The listing builds one solid part. Answer for the finished solid, in the listing's coordinates (mm). Face numbers are marked on the shaded views. Coordinates: 2 decimals unless noted, no trailing zeros. Write each loop counter-clockwise with the first axis right and the second up, starting at its lowest first coordinate (ties: lowest second). Pieces come first, ordered by that corner, then holes.
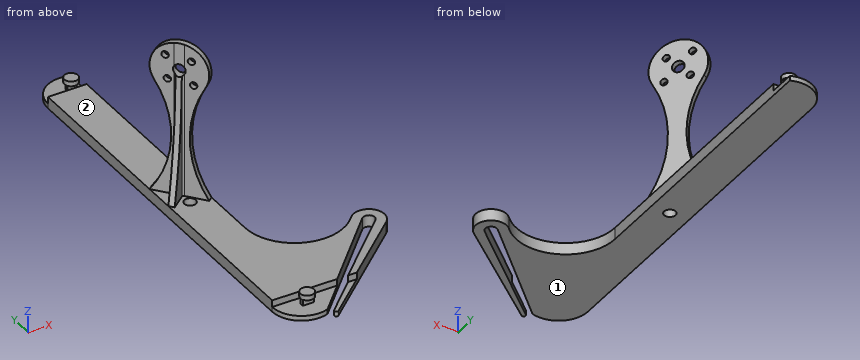
from build123d import *

# Parameters (mm, degrees)
PAD_DEPTH       = 6
SKETCH001_W     = 31.342523
SKETCH001_H     = 18.2690453429
SKETCH001_R     = 2.5
POCKET_DEPTH    = 3.5
SKETCH013_W     = 48.164109
SKETCH013_H     = 19.3260583096
SKETCH013_R     = 3.021402
POCKET008_DEPTH = 3.5
PAD001_DEPTH    = 80
POCKET009_DEPTH = 3
SKETCH015_R     = 3
SKETCH015_R_2   = 1.75
POCKET010_DEPTH = 80.3906309058
POCKET011_DEPTH = 5.5
POCKET012_DEPTH = 3.5
POCKET013_DEPTH = 3.5
SKETCH022_R     = 3.5
PAD002_DEPTH    = 2.5
SKETCH023_R     = 3.5
PAD003_DEPTH    = 2.5
SKETCH024_R     = 3
POCKET014_DEPTH = 6.001


with BuildPart() as part:
    # Sketch → Pad (new body)
    with BuildSketch(Plane.XY):
        with BuildLine():
            Line((148.7359710531, -99.0646793429), (148.7359710531, 92.9353206571))
            ThreePointArc((168.7359710531, 107.0774562808), (155.0757170152, 105.182769371), (148.7359710531, 92.9353206571))
            Line((168.7359710531, -42.6963517772), (168.7359710531, 107.0774562808))
            ThreePointArc((168.7359710531, -42.6963517772), (185.2022873789, -66.5007048599), (213.2847541452, -59.4891530095))
            ThreePointArc((224.5749857013, -70.7793845656), (224.9509601574, -59.1131785534), (213.2847541452, -59.4891530095))
            Line((172.271504959, -116.7423812201), (224.5749857013, -70.7793845656))
            ThreePointArc((170.8572913966, -115.3281676577), (170.8572913966, -116.7423812201), (172.271504959, -116.7423812201))
            Line((170.8572913966, -115.3281676577), (221.4154262515, -66.8913531464))
            ThreePointArc((221.4154262515, -66.8913531464), (221.4154262515, -62.6487124593), (217.1727855643, -62.6487124593))
            Line((168.7359710531, -113.2068473142), (217.1727855643, -62.6487124593))
            ThreePointArc((148.7359710531, -99.0646793429), (155.0757038094, -111.3121510664), (168.7359710531, -113.2068473142))
        make_face()
    extrude(amount=PAD_DEPTH)

    # Sketch001 → Pocket (cut)
    with BuildSketch(Plane.XY.offset(6)):
        with Locations((159.4964165, 102.0698433285)):
            Rectangle(SKETCH001_W, SKETCH001_H)
        with Locations((163.7359710531, 97.9353206571)):
            Circle(SKETCH001_R, mode=Mode.SUBTRACT)
    extrude(amount=-POCKET_DEPTH, mode=Mode.SUBTRACT)

    # Sketch013 → Pocket008 (cut)
    with BuildSketch(Plane.XY.offset(6)):
        with Locations((169.3588635, -108.7277408452)):
            Rectangle(SKETCH013_W, SKETCH013_H)
        with Locations((163.7359710531, -104.0647116904)):
            Circle(SKETCH013_R, mode=Mode.SUBTRACT)
    extrude(amount=-POCKET008_DEPTH, mode=Mode.SUBTRACT)

    # Sketch014 → Pad001 (new body)
    with BuildSketch(Plane.XY.offset(6)):
        with BuildLine():
            Line((148.7359710531, 5.9602104844), (155.9970967848, -3.0092063605))
            ThreePointArc((155.849066174, -4.4156511472), (156.2143657321, -3.7430868972), (155.9970967848, -3.0092063605))
            Line((148.7359710531, -10.174005219), (155.849066174, -4.4156511472))
            Line((148.7359710531, -10.174005219), (150.6235923171, -12.5057183154))
            Line((150.6235923171, -12.5057183154), (157.7366874381, -6.7473642436))
            ThreePointArc((159.1431322249, -6.8953948544), (158.4705679748, -6.5300952963), (157.7366874381, -6.7473642436))
            Line((159.1431322249, -6.8953948544), (166.4042579566, -15.8648116991))
            Line((166.4042579566, -15.8648116991), (168.7359710531, -13.9771904352))
            Line((151.0676841499, 7.8478317492), (168.7359710531, -13.9771904352))
            Line((148.7359710531, 5.9602104844), (151.0676841499, 7.8478317492))
        make_face()
    extrude(amount=PAD001_DEPTH)

    # Sketch016 → Pocket009 (cut)
    with BuildSketch(Plane(origin=(95.0976832559, 76.9856331596, 0), x_dir=(-0.629207088, 0.7772376988, 0), z_dir=(0.7772376988, 0.629207088, 0))):
        with BuildLine():
            ThreePointArc((-90.8226866435, 64.9598793146), (-102.9933476305, 86), (-115.1640086175, 64.9598793146))
            ThreePointArc((-117.0334683159, 6), (-107.9048310085, 35.2201328201), (-115.1640086175, 64.9598793146))
            Line((-117.0334683159, 6), (-129.946838, 10.190964))
            Line((-129.946838, 10.190964), (-129.946838, 98.716408))
            Line((-129.946838, 98.716408), (-69.304048, 98.716408))
            Line((-69.304048, 98.716408), (-45.866948, 9.880296))
            Line((-45.866948, 9.880296), (-88.9532269451, 6))
            ThreePointArc((-90.8226866435, 64.9598793146), (-99.1328607178, 35.18680854), (-88.9532269451, 6))
        make_face()
    extrude(amount=-POCKET009_DEPTH, mode=Mode.SUBTRACT)

    # Sketch015 → Pocket010 (cut, through all)
    with BuildSketch(Plane(origin=(95.0976832559, 76.9856331596, 0), x_dir=(-0.629207088, 0.7772376988, 0), z_dir=(0.7772376988, 0.629207088, 0))):
        with Locations((-102.9933476305, 71.9598793146)):
            Circle(SKETCH015_R)
        with Locations((-96.2758332092, 78.6773937359)):
            Circle(SKETCH015_R_2)
        with Locations((-108.65020188, 77.6167335641)):
            Circle(SKETCH015_R_2)
        with Locations((-109.7108620518, 65.2423648933)):
            Circle(SKETCH015_R_2)
        with Locations((-97.336493381, 66.3030250651)):
            Circle(SKETCH015_R_2)
    extrude(amount=-POCKET010_DEPTH, mode=Mode.SUBTRACT)

    # Sketch017 → Pocket011 (cut, symmetric)
    with BuildSketch(Plane(origin=(63.8603337123, -78.8844559543, 0), x_dir=(-0.7772376988, -0.629207088, 0), z_dir=(-0.629207088, 0.7772376988, 0))):
        with BuildLine():
            ThreePointArc((-118.353410552, 69.3618031032), (-116.0536600062, 37.3521449631), (-109.2016476719, 6.0000000001))
            Line((-98.802281, 97.315555), (-109.2016476718, 6))
            Line((-119.353410552, 97.315555), (-98.802281, 97.315555))
            Line((-119.353410552, 73.6181917099), (-119.353410552, 97.315555))
            Line((-118.353410552, 69.3618031032), (-119.353410552, 73.6181917099))
        make_face()
    extrude(amount=POCKET011_DEPTH, both=True, mode=Mode.SUBTRACT)

    # Sketch020 → Pocket012 (cut)
    with BuildSketch(Plane.XY.offset(6)):
        with BuildLine():
            ThreePointArc((166.0456698843, 98.892029238), (163.7359710531, 100.4353206571), (161.4262722218, 98.892029238))
            Line((161.4262722218, 98.892029238), (166.0456698843, 98.892029238))
        make_face()
        with BuildLine():
            ThreePointArc((161.4262722218, 96.9786120762), (163.7359710531, 95.4353206571), (166.0456698843, 96.9786120762))
            Line((161.4262722218, 96.9786120762), (166.0456698843, 96.9786120762))
        make_face()
    extrude(amount=-POCKET012_DEPTH, mode=Mode.SUBTRACT)

    # Sketch021 → Pocket013 (cut)
    with BuildSketch(Plane.XY.offset(6)):
        with BuildLine():
            ThreePointArc((166.5273825204, -102.9084712025), (163.7359710531, -101.0433096904), (160.9445595858, -102.9084712025))
            Line((160.9445595858, -102.9084712025), (166.5273825204, -102.9084712025))
        make_face()
        with BuildLine():
            ThreePointArc((160.9445595858, -105.2209521783), (163.7359710531, -107.0861136904), (166.5273825204, -105.2209521783))
            Line((160.9445595858, -105.2209521783), (166.5273825204, -105.2209521783))
        make_face()
    extrude(amount=-POCKET013_DEPTH, mode=Mode.SUBTRACT)

    # Sketch022 → Pad002 (new body)
    with BuildSketch(Plane.XY.offset(6)):
        with Locations((163.7359710531, 97.9353206571)):
            Circle(SKETCH022_R)
    extrude(amount=PAD002_DEPTH)

    # Sketch023 → Pad003 (new body)
    with BuildSketch(Plane.XY.offset(6)):
        with Locations((163.7359710531, -104.0647116904)):
            Circle(SKETCH023_R)
    extrude(amount=PAD003_DEPTH)

    # Sketch024 → Pocket014 (cut, through all)
    with BuildSketch(Plane.XY.offset(6)):
        with Locations((158.7359710531, -12.174005219)):
            Circle(SKETCH024_R)
    extrude(amount=-POCKET014_DEPTH, mode=Mode.SUBTRACT)


solid = part.part
1. Section A-A on x = 177 is taken. Give the vertices of the cut face in (y, z), then the cut area to 3 significant figures.
Results found:
outline: (-112.59, 0) - (-109.44, 0) - (-109.44, 2.5) - (-112.59, 2.5) - close; (-104.58, 0) - (-61.46, 0) - (-61.46, 6) - (-99.06, 6) - (-99.06, 2.5) - (-104.58, 2.5) - close
area: 247 mm2
2. Section D-D on x = 207 is taken. Give the vertices of the cut face in (y, z), then the cut area to 3 significant figures.
Results found:
outline: (-86.22, 0) - (-80.7, 0) - (-80.7, 6) - (-86.22, 6) - close; (-73.27, 0) - (-64.67, 0) - (-64.67, 6) - (-73.27, 6) - close
area: 84.7 mm2
3. For a pull along Y with two mould halves and no side action, classify the marked faces 1 and 2 as pulls with the +Y half, pulls with the -Y half, needs draft (parallel to the pull), parting line crosses it, or undercut.
Results found:
face 1: needs draft
face 2: undercut
4. Find the intervals of material crossed by L1, parallel to X at y = 60, z = 5.5; L2, parallel to Y at x = 154.5, z = 23; L3, parallel to Y at x = 156, z = 43, in increasing order.
Results found:
L1: x = 148.74 to 168.74
L2: y = -9.37 to -5.51, -1.16 to -0.08
L3: y = -7.08 to -4.26, -3.01 to -0.81
5. Section B-B on z = 42 is taken. Give the vertices of the cut face in (x, y), then the cut area to 3 significant figures.
Results found:
outline: (154.54, -5.47) - (156.43, -7.8) - (157.74, -6.75) arc R1 cw to (159.14, -6.9) - (160.78, -8.92) - (163.11, -7.03) - (157.33, 0.12) - (154.99, -1.77) - (156, -3.01) arc R1 cw to (155.85, -4.42) - close
area: 36.0 mm2
6. Section C-C on y = -77 is taken. Give the vertices of the cut face in (x, z), then the cut area to 3 significant figures.
Results found:
outline: (148.74, 0) - (203.42, 0) - (203.42, 6) - (148.74, 6) - close; (210.86, 0) - (217.5, 0) - (217.5, 6) - (210.86, 6) - close
area: 368 mm2
7. Flat-ended cylindrical pins translate along their axes: P1, Ø6, axis at x = 154, y = 0, coming from the +Z side; P2, Ø2, axis at x = 164.5, y = -104, coming from the +Z side; P3, Ø3, axis at x = 158.5, z = 45, coming from the -Y side. Find the tip coordinate at first contact, or state that the pin passes through.
Results found:
P1: stops at z = 85.65
P2: stops at z = 8.5
P3: stops at y = -7.95
